Build history of the part. All positions in model axes, mm. A direction names the side the tool comes from. Give positions to 0.01 mm unless a question says otherwise; leave off trailing zeros. Order: outer loops, then holes, each group sorted by start corner. A loop starts at its lowest first (then second) coordinate and runs counter-clockwise, first axis right, second up. Notation, with made-up numbers: M 62.5,67 L 76.5,67 A9 ccw 76.5,73 Z; hole C -8.75,-1.75 d9. An arc over 180 degrees is marked long. Use CSV: the item, a comma, the result in double quotes. Start each with the question number.
Item 1: Band-saw the part on A-A on x = 11.5. Write the cut outline in (y, z), plus the area to 3 significant figures.
Item 2: Pin check, flat tips, straight feed: P1, Ø12, axis at x = -18, z = 855.5, coming from the +Y side; P2, Ø25, axis at x = 0, z = 370, coming from the -Y side; P3, Ø25, axis at x = -12, y = -103.5, coming from the +Z side. Stop position of each tip, or through.
Item 3: Band-saw the part on B-B on z = 720.5. Write the cut outline in (x, y), plus the area to 3 significant figures.
Item 4: Wall check: line 1 along Y through (x, z) = (-12, 176.5); line 2 along Y through (x, z) = (-5.5, 851.5); line 3 along Z through (x, y) = (7, -142). Give the ranges that are in metal, low to high.
Item 5: Which spindle directions (+Z, -Z, +X, -X, +Y, -Y) get a long thin tool onto all of the face, cutting with end or side? Do faces 1 (the flat face through (0, 175, 200)), 2 (the flat face through (0, 150, 99)), 3 (the flat face through (0, -175, 200)), 4 (the flat face through (0, -3, -50)). Say none if no direction does.
Item 6: Band-saw the part on C-C on y = -81. Write the cut outline in (x, z), plus the area to 3 significant figures.
Item 7: Two-plate mould, pull along Y, no slides. Class faces 5 (the flat face through (0, -200, 73)), 6 (the flat face through (0, 0, 1000)), 7 (the flat face through (0, -25, 493)): pulls with the +Y half, pulls with the -Y half, needs draft (parallel to the pull), parting line crosses it, or undercut.
from build123d import *

# Parameters (mm, degrees)
F0_W          = 50
F0_H          = 50
F1_DEPTH      = 1000
F2_W          = 200
F2_H          = 50
F3_DEPTH      = 25
F3_DEPTH_BACK = 25
F4_W          = 50
F4_H          = 200
F5_DEPTH      = 25
F5_DEPTH_BACK = 25


with BuildPart() as f1:
    # F0 (on Top) → F1 (new body)
    with BuildSketch(Plane.XY):
        Rectangle(F0_W, F0_H)
    extrude(amount=F1_DEPTH)

    # F2 (on Right) → F3 (join, two sides)
    with BuildSketch(Plane.YZ) as f3_sk:
        with Locations((-100, -25)):
            Rectangle(F2_W, F2_H)
        with Locations((100, -25)):
            Rectangle(F2_W, F2_H)
    extrude(amount=F3_DEPTH)
    extrude(f3_sk.sketch, amount=-F3_DEPTH_BACK)

    # F4 (on Right) → F5 (join, two sides)
    with BuildSketch(Plane.YZ) as f5_sk:
        with Locations((175, 100)):
            Rectangle(F4_W, F4_H)
        with Locations((-175, 100)):
            Rectangle(F4_W, F4_H)
    extrude(amount=F5_DEPTH)
    extrude(f5_sk.sketch, amount=-F5_DEPTH_BACK)


solid = f1.part
Model answer:
1,outline,"M -200,-50 L 200,-50 L 200,200 L 150,200 L 150,0 L 25,0 L 25,1000 L -25,1000 L -25,0 L -150,0 L -150,200 L -200,200 Z"
1,area,"90,000 mm^2"
2,P1,"stops at y = 25"
2,P2,"stops at y = -25"
2,P3,"stops at z = 0"
3,outline,"M -25,-25 L 25,-25 L 25,25 L -25,25 Z"
3,area,"2,500 mm^2"
4,line 1,"y = -200 to -150, -25 to 25, 150 to 200"
4,line 2,"y = -25 to 25"
4,line 3,"z = -50 to 0"
5,face 1,"+Z, +X, -X, +Y"
5,face 2,"+Z, +X, -X"
5,face 3,"+Z, +X, -X, -Y"
5,face 4,"-Z, +X, -X, +Y, -Y"
6,outline,"M -25,-50 L 25,-50 L 25,0 L -25,0 Z"
6,area,"2,500 mm^2"
7,face 5,"pulls with the -Y half"
7,face 6,"needs draft"
7,face 7,"undercut"
